The figure shows three views and two pictorial views of one solid part (mm, origin at its lowest corner). Answer the questions. A direction names the side the tool comes from. Coordinates: 2 decimals unless noted, no trailing zeros. Order: outer loops, then holes, each group sorted by start corner. A loop starts at its lowest first (then second) coordinate and runs counter-clockwise, first axis right, second up. Notation, with made-up numbers: (59.25, 51) -> (112.25, 51) arc R30 cw to (112.25, 83) -> close; hole circle Ø6 at (6, -5). An arc over 180 degrees is marked (long way). Return JSON: item names as keys, results as strings.
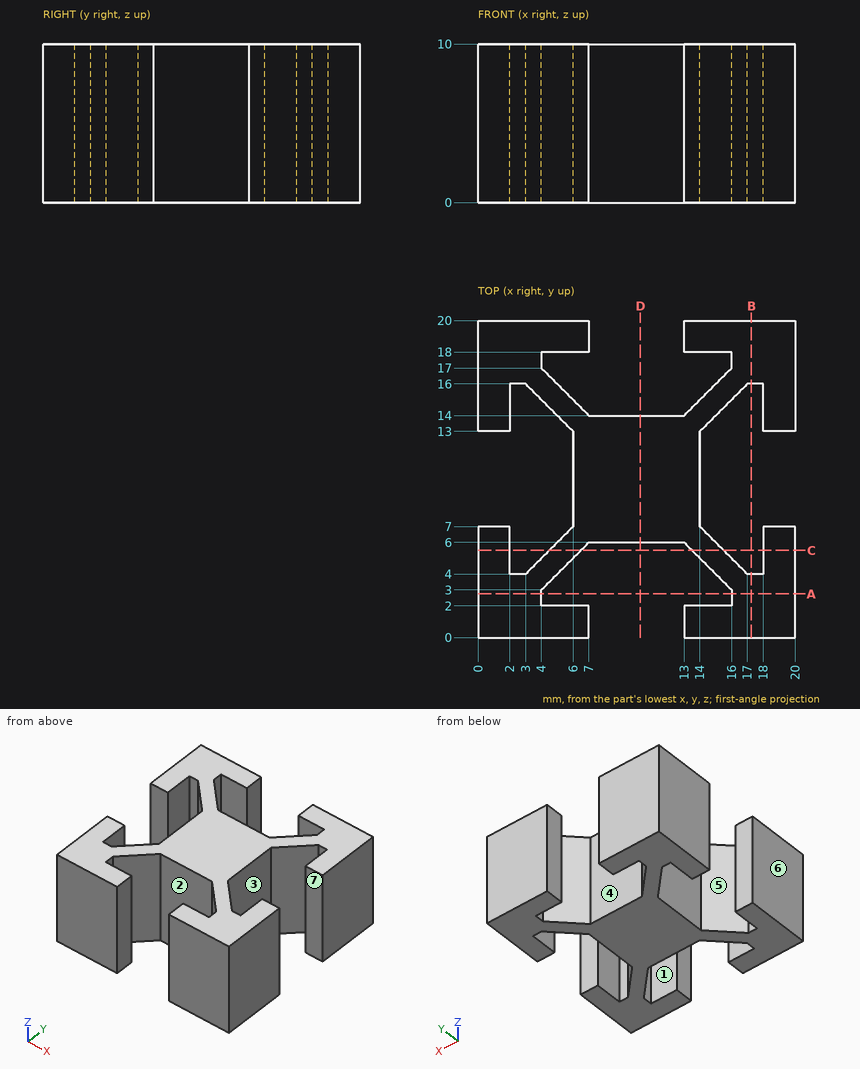
1. For the marked faces 1, 2, 3 and 4, determine the directions among +Z, -Z, +X, -X, +Y, -Y from which every point of the face is accessible in a straight line to the end or side of a thin tool.
Answer block:
{"face 1": "+Z, -Z", "face 2": "+Z, -Z, -Y", "face 3": "+Z, -Z, +X", "face 4": "+Z, -Z, +Y"}
2. This flat-tipped pin is pushed along its axis until it touches: pin 1 Ø1.8 at (y, z) = (10, 7) entering from +X. Where does it stop, or does it pass through?
Answer block:
{"pin 1": "stops at x = 14"}
3. The part is cut by section A-A on y = 2.75. Give the vertices of the cut face in (x, z), and give its area (3 significant figures).
Answer block:
{"outline": "(0, 0) -> (4, 0) -> (4, 10) -> (0, 10) -> close; (16, 0) -> (20, 0) -> (20, 10) -> (16, 10) -> close", "area": "80.0 mm2"}
4. The part is cut by section D-D on x = 10.25. Give the vertices of the cut face in (y, z), and give its area (3 significant figures).
Answer block:
{"outline": "(6, 0) -> (14, 0) -> (14, 10) -> (6, 10) -> close", "area": "80.0 mm2"}
5. Consider line 1 (Y direction, x = 1.75, z = 1); line 2 (X direction, y = 17.75, z = 4). Determine where each line is inside the solid, lowest interval first. Write a range as from..to.
Answer block:
{"line 1": "y = 0..7, 13..20", "line 2": "x = 0..4, 16..20"}
6. Determine the mould class of the marked faces 5, 6 and 7 for opening direction X: pulls with the +X half, pulls with the -X half, needs draft (parallel to the pull), parting line crosses it, or undercut.
Answer block:
{"face 5": "undercut", "face 6": "pulls with the -X half", "face 7": "needs draft"}
7. The part is cut by section C-C on y = 5.5. Give the vertices of the cut face in (x, z), and give its area (3 significant figures).
Answer block:
{"outline": "(0, 0) -> (2, 0) -> (2, 10) -> (0, 10) -> close; (4.5, 0) -> (6.5, 0) -> (6.5, 10) -> (4.5, 10) -> close; (13.5, 0) -> (15.5, 0) -> (15.5, 10) -> (13.5, 10) -> close; (18, 0) -> (20, 0) -> (20, 10) -> (18, 10) -> close", "area": "80.0 mm2"}
